Solid Edge part; units mm, degrees
sketch "Sketch1" plane through (0, 0, 0) normal (0, -1, 0) x (1, 0, 0)
  line L0 (5.0412, 10) -> (5.0412, 32.6352)
  line L1 (5.0412, 32.6352) -> (11.1303, 30.9718)
  line L2 (11.1303, 30.9718) -> (2.809, 40.9718)
  line L3 (0, 40.9718) -> (2.809, 40.9718)
  line L4 (0, 0) -> (0, 40.9718)
  line L5 (0, 0) -> (0.0508, 0)
  line L6 (0.0508, 0) -> (5.0412, 0)
  line L7 (5.0412, 0) -> (5.0412, 10)
extrude "Protrusion1" add sketch "Sketch1" against normal blind 15
sketch "Sketch2" plane through (0, 0, 0) normal (0, -1, 0) x (1, 0, 0)
  line L0 (-1.4115, 10) -> (-1.4115, 1)
  line L1 (0.1393, 10) -> (-1.4115, 10)
  line L2 (0.1393, -0.0543) -> (0.1393, 10)
  line L3 (-5.8107, -0.0543) -> (0.1393, -0.0543)
  line L4 (-5.8107, 9.9052) -> (-5.8107, -0.0543)
  line L5 (-3.9551, 9.9052) -> (-5.8107, 9.9052)
  line L6 (-3.9551, 0.9052) -> (-3.9551, 9.9052)
  line L7 (-1.4115, 0.9052) -> (-3.9551, 0.9052)
extrude "ProtrusioneEstrusa_8" add sketch "Sketch2" against normal blind 50 material side at (-1.4615, 0, 5.5)
sketch "Sketch3" plane through (3.7254, 22.5, 10) normal (0, 0, 1) x (0, 1, 0)
  line L0 (-2.0677, 7.6805) -> (-6.3668, 7.6805)
  line L1 (-6.3668, 7.6805) -> (-6.3668, 3.0032)
  line L2 (-6.3668, 3.0032) -> (-2.0677, 3.0032)
  line L3 (-2.0677, 3.0032) -> (-2.0677, 7.6805)
extrude "Cutout1" cut sketch "Sketch3" against normal blind 8.8165
sketch "Sketch4" plane through (3.7254, 22.5, 10) normal (0, 0, 1) x (0, 1, 0)
  line L0 (-2.0677, 3.0032) -> (-2.0677, 7.6805)
  line L1 (-2.0677, 7.6805) -> (-6.3668, 7.6805)
  line L2 (-6.3668, 7.6805) -> (-6.3668, 3.0032)
  line L3 (-6.3668, 3.0032) -> (-2.0677, 3.0032)
extrude "Cutout2" cut sketch "Sketch4" against normal up to vertex (9.0948 mm away)
sketch "Sketch5" plane through (3.7254, 22.5, 10) normal (0, 0, 1) x (0, 1, 0)
  line L0 (-1.0199, 4.0793) -> (-2.0677, 4.0793)
  line L1 (-2.0677, 3.0032) -> (-2.0677, 4.0793)
  line L2 (-6.3668, 3.0032) -> (-2.0677, 3.0032)
  line L3 (-6.3668, 4.0793) -> (-6.3668, 3.0032)
  line L4 (-6.3668, 4.0793) -> (-7.3668, 4.0793)
  line L5 (-7.3668, 4.0793) -> (-7.3668, 0.7486)
  line L6 (-7.3668, 0.7486) -> (-1.0199, 0.7486)
  line L7 (-1.0199, 0.7486) -> (-1.0199, 4.0793)
extrude "Protrusion2" add sketch "Sketch5" against normal up to vertex (10.0543 mm away)
sketch "Sketch6" plane through (1.2976, 7.5, 40.9718) normal (0, 0, 1) x (0, -1, 0)
  line L0 (7.5, 1.5113) -> (-7.479, 1.2818)
  line L1 (-7.479, 1.2818) -> (-7.479, -7.1083)
  line L2 (-7.479, -7.1083) -> (7.5, -7.1083)
  line L3 (7.5, -7.1083) -> (7.5, 1.5113)
extrude "Protrusion3" add sketch "Sketch6" against normal up to vertex (41.026 mm away)
fillet "Rotondo_2" radius 2 1 edges at (5.0412, 7.5, 32.6352)
fillet "Rotondo_3" radius 10 1 edges at (-5.8107, 7.4895, 40.9718)
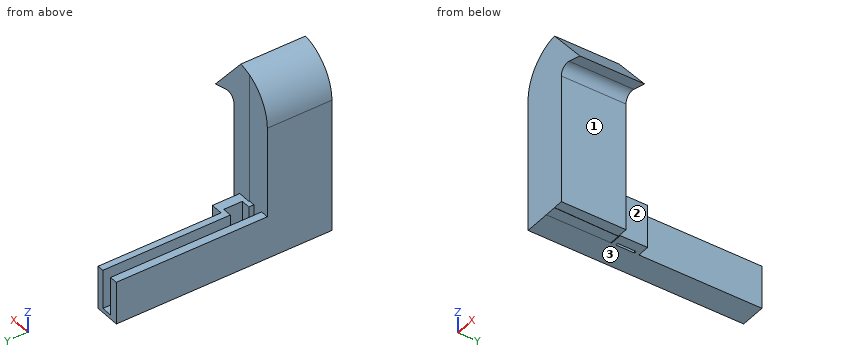
Here's how the part is built. I have some questions about the finished solid (model axes, mm). Face numbers are marked on the shaded views. A direction names the side the tool comes from. Give positions to 0.01 mm unless a question says otherwise; leave off trailing zeros. Order: outer loops, then holes, each group sorted by start corner. A loop starts at its lowest first (then second) coordinate and runs counter-clockwise, first axis right, second up. Notation, with made-up numbers: (88.25, 86.5) -> (144.25, 86.5) arc R10 ccw to (144.25, 94.5) -> close; hole circle Ø3 at (-34.75, -23.5). An arc over 180 degrees is marked (long way). Use a Markdown table: item, result. Add a question column.
Item 1: Imagine slicing it at D-D on x = -4.5. Please give me the cut outline in (y, z).
Item 2: Will these pins go through, and if not, where does the flat tip stop? pin 1 (1.5 mm diameter, centred on y = 20, z = 10, fed in from -X); pin 2 (8 mm diameter, centred on y = 11, z = 5, fed in from +X); pin 3 (3 mm diameter, centred on y = 19, z = 4, fed in from +X); pin 4 (1.5 mm diameter, centred on x = -4.5, y = 29, fed in from +Z).
Item 3: Imagine slicing it at A-A on y = 30.5. Please give me the cut outline in (x, z), plus the area to 3 significant figures.
Item 4: For the marked faces 1, 2 and 3, which set-ups out of +Z, -Z, +X, -X, +Y, -Y let a thin tool reach every point of the face, with its end or its side?
Item 5: Imagine slicing it at C-C on z = 7.5. Please give me the cut outline in (x, y).
Item 6: I need wall thicknesses on line 1 (X direction, y = 45.5, z = 9.5); line 2 (Z direction, x = -0.5, y = 41); line 3 (Y direction, x = 7.5, z = 34). Which ranges of each line are inside material? Lowest first, please.
Data:
| question | item | result |
|---|---|---|
| 1 | outline | (0, -0.05) -> (50, -0.05) -> (50, 9.91) -> (14.98, 9.91) -> (14.98, 36.02) -> (0, 36.02) -> close |
| 2 | pin 1 | stops at x = -5.81 |
| 2 | pin 2 | stops at x = 5.04 |
| 2 | pin 3 | stops at x = 2.98 |
| 2 | pin 4 | stops at z = 9.91 |
| 3 | outline | (-5.81, -0.05) -> (0.14, -0.05) -> (0.14, 10) -> (-1.41, 10) -> (-1.41, 0.91) -> (-3.96, 0.91) -> (-3.96, 9.91) -> (-5.81, 9.91) -> close |
| 3 | area | 36.5 mm² |
| 4 | face 1 | -Z, +X, +Y, -Y |
| 4 | face 2 | +Z, -Z, +X, +Y |
| 4 | face 3 | -Z, +X, -X, +Y, -Y |
| 5 | outline | (-5.81, 0) -> (5.04, 0) -> (5.04, 15) -> (0.14, 15) -> (0.14, 15.13) -> (2.98, 15.13) -> (2.98, 21.48) -> (0.14, 21.48) -> (0.14, 50) -> (-1.41, 50) -> (-1.41, 20.43) -> (0.72, 20.43) -> (0.72, 16.13) -> (-1.41, 16.13) -> (-1.41, 14.98) -> (-3.96, 14.98) -> (-3.96, 50) -> (-5.81, 50) -> close |
| 6 | line 1 | x = -5.81 to -3.96, -1.41 to 0.14 |
| 6 | line 2 | z = -0.05 to 10 |
| 6 | line 3 | y = 0 to 15 |
